Can you work these out from the model? Positions are in its coordinate system, mm. Coordinates: 2 decimals unless noted, no trailing zeros. Loops run counter-clockwise (first coordinate to the right, second up) from the corner with the lowest first, then second, coordinate; pieces in that order, holes last.
```python
from build123d import *

# Parameters (mm, degrees)
PAD_DEPTH       = 3
PAD001_DEPTH    = 3
FILLET_R        = 3
FILLET001_R     = 1
FILLET002_R     = 1
SKETCH003_W     = 1.5
SKETCH003_H     = 14
SKETCH003_H_2   = 4
SKETCH003_W_2   = 40.5
SKETCH003_H_3   = 1.5
PAD002_DEPTH    = 1
SKETCH004_R     = 1.55
POCKET_DEPTH    = 3.001
SKETCH005_W     = 14
SKETCH005_H     = 26
SKETCH005_W_2   = 26.4
SKETCH005_H_2   = 10
POCKET001_DEPTH = 3.001
FILLET003_R     = 1


with BuildPart() as part:
    # Sketch → Pad (new body)
    with BuildSketch(Plane.XY):
        Polygon((0, 3), (51, 3), (51, 0), (46.5, 0), (46.5, -20), (48.5, -20), (48.5, -36), (0, -36), align=None)
    extrude(amount=PAD_DEPTH)

    # Sketch001 (on Face10 of Pad) → Pad001 (join)
    with BuildSketch(Plane.XY.offset(3)):
        with BuildLine():
            Line((46.5, 6), (46.5, 3))
            Line((46.5, 3), (40.5, 3))
            Line((40.5, 3), (40.5, 6))
            ThreePointArc((46.5, 6), (43.5, 9), (40.5, 6))
        make_face()
    extrude(amount=-PAD001_DEPTH)

    # Fillet
    fillet_edges = [part.edges().sort_by_distance(p)[0] for p in [
        (48.5, -36, 1.5),
    ]]
    fillet(fillet_edges, radius=FILLET_R)

    # Fillet001
    fillet001_edges = [part.edges().sort_by_distance(p)[0] for p in [
        (48.5, -20, 1.5),
    ]]
    fillet(fillet001_edges, radius=FILLET001_R)

    # Fillet002
    fillet002_edges = [part.edges().sort_by_distance(p)[0] for p in [
        (51, 3, 1.5),
        (51, 0, 1.5),
    ]]
    fillet(fillet002_edges, radius=FILLET002_R)

    # Sketch003 → Pad002 (join)
    with BuildSketch(Plane(origin=(0, 0, 0), x_dir=(1, 0, 0), z_dir=(0, 0, -1))):
        with Locations((42.55, 9)):
            Rectangle(SKETCH003_W, SKETCH003_H)
        with Locations((44.55, 26)):
            Rectangle(SKETCH003_W, SKETCH003_H_2)
        with Locations((20.25, 32.05)):
            Rectangle(SKETCH003_W_2, SKETCH003_H_3)
    extrude(amount=PAD002_DEPTH)

    # Sketch004 (on Face1 of Pad002) → Pocket (cut, through all)
    with BuildSketch(Plane(origin=(0, 0, 0), x_dir=(1, 0, 0), z_dir=(0, 0, -1))):
        with Locations((45.5, 33)):
            Circle(SKETCH004_R)
        with Locations((43.5, -6)):
            Circle(SKETCH004_R)
    extrude(amount=-POCKET_DEPTH, mode=Mode.SUBTRACT)

    # Mirrored: part across YZ


with BuildPart() as part_1:
    add(part.part)
    add(part.part.mirror(Plane.YZ))

    # Sketch005 (on Face14 of Mirrored) → Pocket001 (cut, through all)
    with BuildSketch(Plane(origin=(0, 0, 0), x_dir=(1, 0, 0), z_dir=(0, 0, -1))):
        with Locations((-31.3, 10)):
            Rectangle(SKETCH005_W, SKETCH005_H)
        with Locations((-10, 18)):
            Rectangle(SKETCH005_W_2, SKETCH005_H_2)
    extrude(amount=-POCKET001_DEPTH, mode=Mode.SUBTRACT)

    # Fillet003
    fillet003_edges = [part_1.edges().sort_by_distance(p)[0] for p in [
        (-24.3, 3, 1.5),
        (-38.3, 3, 1.5),
        (-38.3, -23, 1.5),
        (-23.2, -23, 1.5),
        (-23.2, -13, 1.5),
        (3.2, -13, 1.5),
        (3.2, -23, 1.5),
        (-24.3, -23, 1.5),
    ]]
    fillet(fillet003_edges, radius=FILLET003_R)


solid = part_1.part
```
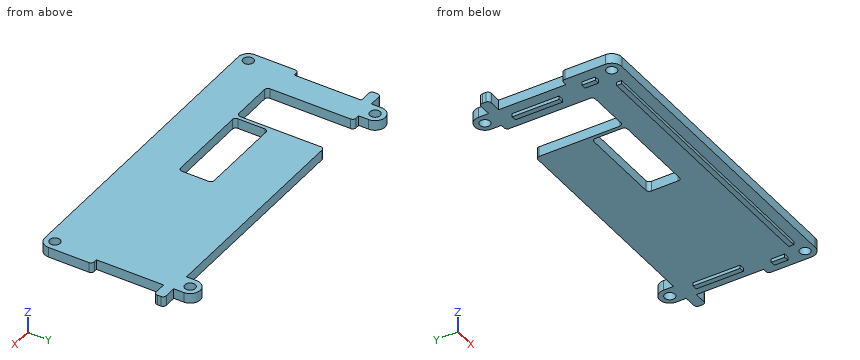
Item 1: I'm going to push flat-ended pins straight in: P1, Ø0.9, axis at y = -10, z = 1, coming from the -X side; P2, Ø4, axis at x = 45.5, y = -33, coming from the -Z side; P3, Ø0.5, axis at x = -42, z = -0.5, coming from the +Y side. Where does each tip first touch, or does it pass through?
Results are:
P1: stops at x = -46.5
P2: stops at z = 0
P3: stops at y = -2
Item 2: I need wall thicknesses on line 1 along X through (y, z) = (-33, 1.1); line 2 along X through (y, z) = (6, 1.7); line 3 along Y through (x, z) = (-43.5, 2.05). Which ranges of each line are inside material? Lowest first, please.
Results are:
line 1: x = -48.5 to -47.05, -43.95 to 43.95, 47.05 to 48.5
line 2: x = -46.5 to -45.05, -41.95 to -40.5, 40.5 to 41.95, 45.05 to 46.5
line 3: y = -36 to 4.45, 7.55 to 9
Item 3: Suppose I cut it at B-B, the plane z = 1.3. Count the separate pieces of the cut face and the enclosed holes in it, plus the area to 3 significant figures.
Results are:
separate pieces: 1
enclosed holes: 5
area: 3,120 mm2
Item 4: Suppose I cut it at A-A, the plane x = -2. Please give me the cut outline in (y, z).
Results are:
outline: (-36, 0) - (-32.8, 0) - (-32.8, -1) - (-31.3, -1) - (-31.3, 0) - (-23, 0) - (-23, 3) - (-36, 3) - close; (-13, 0) - (3, 0) - (3, 3) - (-13, 3) - close
